from build123d import *

# Parameters (mm, degrees)
F0_W     = 2.7374038473
F0_H     = 4.5464726281
F1_DEPTH = 3


with BuildPart() as f1:
    # F0 (on Front) → F1 (new body)
    with BuildSketch(Plane.XZ):
        with BuildLine():
            Line((-13.9879264009, 8.4983842463), (-10.7078288449, 8.4983842463))
            ThreePointArc((-10.7078288449, 8.4983842463), (-12.3096819162, -5.9457433928), (0, -13.6704108706))
            Line((0, -13.6704108706), (29.832560569, -13.6704108706))
            ThreePointArc((29.832560569, -13.6704108706), (41.0439649972, -7.8220549805), (42.6626390029, 4.7190275219))
            ThreePointArc((42.6626390029, 4.7190275219), (52.7277631814, 0.6811115523), (57.2114773095, -9.193492122))
            Line((57.2114773095, -9.193492122), (57.2114773095, 27.5829305145))
            ThreePointArc((57.2114773095, 27.5829305145), (52.7277631814, 17.7083268402), (42.6626390029, 13.6704108706))
            Line((42.6626390029, 13.6704108706), (29.832560569, 13.6704108706))
            Line((29.832560569, 13.6704108706), (0, 13.6704108706))
            Line((0, 13.6704108706), (-14.4307379611, 13.6704108706))
            Line((-14.4307379611, 13.6704108706), (-14.8297163701, 14.5122008398))
            Line((-14.8297163701, 14.5122008398), (-15.268201828, 14.5122008398))
            ThreePointArc((-15.268201828, 14.5122008398), (-15.9753086092, 14.219307621), (-16.268201828, 13.5122008398))
            Line((-16.268201828, 13.5122008398), (-16.268201828, 9.0994058373))
            ThreePointArc((-16.268201828, 9.0994058373), (-15.9753086092, 8.3922990562), (-15.268201828, 8.0994058373))
            Line((-15.268201828, 8.0994058373), (-14.8297163701, 8.0994058373))
            Line((-14.8297163701, 8.0994058373), (-13.9879264009, 8.4983842463))
        make_face()
        with Locations((-10.5523099191, -3.12910098)):
            Rectangle(F0_W, F0_H, mode=Mode.SUBTRACT)
        with BuildLine():
            add(Edge.make_bspline(
                [(8.4533115607, 7.9434605246), (6.0766133419, 9.056249864), (3.699915123, 9.056249864)],
                knots=[0, 0, 0, 1, 1, 1], degree=2))
            add(Edge.make_bspline(
                [(3.699915123, 9.056249864), (0.2516419847, 9.056249864), (-1.7449676943, 6.7596907952)],
                knots=[0, 0, 0, 1, 1, 1], degree=2))
            add(Edge.make_bspline(
                [(-1.7449676943, 6.7596907952), (-3.7415773734, 4.4631317263), (-3.7415773734, 0.4699123682)],
                knots=[0, 0, 0, 1, 1, 1], degree=2))
            add(Edge.make_bspline(
                [(-3.7415773734, 0.4699123682), (-3.7415773734, -3.6332121098), (-1.8159480843, -5.8748186187)],
                knots=[0, 0, 0, 1, 1, 1], degree=2))
            add(Edge.make_bspline(
                [(-1.8159480843, -5.8748186187), (0.1096812048, -8.1164251276), (3.672438843, -8.1164251276)],
                knots=[0, 0, 0, 1, 1, 1], degree=2))
            add(Edge.make_bspline(
                [(3.672438843, -8.1164251276), (5.861382482, -8.1164251276), (8.6685424206, -7.328771768)],
                knots=[0, 0, 0, 1, 1, 1], degree=2))
            Line((8.6685424206, -7.328771768), (8.6685424206, -9.458183467))
            add(Edge.make_bspline(
                [(8.6685424206, -9.458183467), (6.4933369217, -10.2778924866), (3.3015090632, -10.2778924866)],
                knots=[0, 0, 0, 1, 1, 1], degree=2))
            add(Edge.make_bspline(
                [(3.3015090632, -10.2778924866), (-1.3190853545, -10.2778924866), (-3.8308752833, -7.4707325479)],
                knots=[0, 0, 0, 1, 1, 1], degree=2))
            add(Edge.make_bspline(
                [(-3.8308752833, -7.4707325479), (-6.3426652121, -4.6635726093), (-6.3426652121, 0.5019680282)],
                knots=[0, 0, 0, 1, 1, 1], degree=2))
            add(Edge.make_bspline(
                [(-6.3426652121, 0.5019680282), (-6.3426652121, 3.7350103066), (-5.1337088927, 6.1666610854)],
                knots=[0, 0, 0, 1, 1, 1], degree=2))
            add(Edge.make_bspline(
                [(-5.1337088927, 6.1666610854), (-3.9247525733, 8.5983118643), (-1.6419316444, 9.9148836136)],
                knots=[0, 0, 0, 1, 1, 1], degree=2))
            add(Edge.make_bspline(
                [(-1.6419316444, 9.9148836136), (0.6408892845, 11.231455363), (3.731970783, 11.231455363)],
                knots=[0, 0, 0, 1, 1, 1], degree=2))
            add(Edge.make_bspline(
                [(3.731970783, 11.231455363), (7.0199656214, 11.231455363), (9.4836720602, 10.0316578036)],
                knots=[0, 0, 0, 1, 1, 1], degree=2))
            Line((9.4836720602, 10.0316578036), (8.4533115607, 7.9434605246))
        make_face(mode=Mode.SUBTRACT)
        with Locations((-10.5523099191, 3.0826488801)):
            Rectangle(F0_W, F0_H, mode=Mode.SUBTRACT)
        Polygon((24.8978651327, -9.9893915467), (13.2341842784, -9.9893915467), (13.2341842784, 10.9337956631), (15.6658350572, 10.9337956631), (15.6658350572, -7.7867097678), (24.8978651327, -7.7867097678), align=None, mode=Mode.SUBTRACT)
        Polygon((28.2316537711, 10.9337956631), (33.7727035684, 0.4699123682), (39.3503884057, 10.9337956631), (41.9835319044, 10.9337956631), (34.9999774078, -1.8747301906), (34.9999774078, -9.9893915467), (32.540850349, -9.9893915467), (32.540850349, -1.9892146906), (25.5710339924, 10.9337956631), align=None, mode=Mode.SUBTRACT)
    extrude(amount=F1_DEPTH)


solid = f1.part
Could you check a few things on this model? Use its own coordinates, in mm. A direction names the side the tool comes from. Coordinates: 2 decimals unless noted, no trailing zeros. Order: outer loops, then holes, each group sorted by start corner. A loop starts at its lowest first (then second) coordinate and runs counter-clockwise, first axis right, second up.
Q1. Which directions (+Z, -Z, +X, -X, +Y, -Y) give clear straight access to the entire face, cutting with the end or side of a thin tool? Please do faces 5 (the flat face through (57.211, -1, 9)), 6 (the flat face through (24.898, -1, -9)).
Q2. Suppose I cut it at A-A on x = 16.5. Please give me the cut outline in (y, z).
Q3. Thinking about a two-plate mould opening in Z: for faces 1 (the flat face through (20, -3, 3)), 2 (the flat face through (32.541, -1, -6)), 3 (the flat face through (15, -1, -13.67)), 4 (the flat face through (15, -1, 13.67)), which applies, released by +Z, released by -Z, zero draft, split by the parting line, or undercut?
Q4. Will these pins go through, and if not, where does the flat tip stop? pin 1 (0.8 mm diameter, centred on x = -10, y = -2, fed in from -Z); pin 2 (0.8 mm diameter, centred on x = 40.5, y = -1, fed in from -Z); pin 3 (0.9 mm diameter, centred on x = 25.5, y = -1, fed in from +Z).
Q5. Please list where these lines run through material, in increasing order: L1, parallel to Z at x = 23, y = -2.7; L2, parallel to X at y = -0.15, z = -4.5; L3, parallel to X at y = -1.45, z = 6.
Q6. Suppose I cut it at B-B on y = -2.35. Give the number of separate pieces and of enclosed holes in the cut face, and give its area (3 significant figures).
Answer:
1. face 5: +Z, -Z, +X, +Y, -Y
1. face 6: +Y, -Y
2. outline: (-3, -13.67) - (0, -13.67) - (0, -9.99) - (-3, -9.99) - close; (-3, -7.79) - (0, -7.79) - (0, 13.67) - (-3, 13.67) - close
3. face 1: zero draft
3. face 2: undercut
3. face 3: released by -Z
3. face 4: released by +Z
4. pin 1: stops at z = -9.73
4. pin 2: stops at z = -9.03
4. pin 3: stops at z = 13.67
5. L1: z = -13.67 to -9.99, -7.79 to 13.67
5. L2: x = -12.91 to -11.92, -9.18 to -5.57, -2.73 to 13.23, 15.67 to 32.54, 35 to 42.74, 56.21 to 57.21
5. L3: x = -12.28 to -5.21, -2.32 to 13.23, 15.67 to 28.23, 30.84 to 36.72, 39.29 to 57.21
6. separate pieces: 1
6. enclosed holes: 5
6. area: 1,430 mm2
